```python
from build123d import *

# Parameters (mm, degrees)
ESQUISSE1_W             = 100
ESQUISSE1_H             = 100
BOSS_EXTRU_1_DEPTH      = 5
ESQUISSE2_W             = 20
ESQUISSE2_H             = 5
ENL_V_MAT_EXTRU_1_DEPTH = 142.509716981
ESQUISSE3_W             = 2.886751346
ESQUISSE3_H             = 18
ENL_V_MAT_EXTRU_2_DEPTH = 142.509716981
ENL_V_MAT_EXTRU_5_DEPTH = 18
ENL_V_MAT_EXTRU_6_DEPTH = 18
ENL_V_MAT_EXTRU_7_DEPTH = 18
ENL_V_MAT_EXTRU_8_DEPTH = 18


with BuildPart() as part:
    # Esquisse1 → Boss.-Extru.1 (new body)
    with BuildSketch(Plane.XY):
        with Locations((-50, -50)):
            Rectangle(ESQUISSE1_W, ESQUISSE1_H)
    extrude(amount=BOSS_EXTRU_1_DEPTH)

    # Esquisse2 → Enlèv. mat.-Extru.1 (cut, through all)
    with BuildSketch(Plane.XY.offset(5)):
        with Locations((-70, -2.5)):
            Rectangle(ESQUISSE2_W, ESQUISSE2_H)
        with Locations((-30, -2.5)):
            Rectangle(ESQUISSE2_W, ESQUISSE2_H)
        with Locations((-30, -97.5)):
            Rectangle(ESQUISSE2_W, ESQUISSE2_H)
        with Locations((-70, -97.5)):
            Rectangle(ESQUISSE2_W, ESQUISSE2_H)
    extrude(amount=-ENL_V_MAT_EXTRU_1_DEPTH, mode=Mode.SUBTRACT)

    # Esquisse3 → Enlèv. mat.-Extru.2 (cut, through all)
    with BuildSketch(Plane.XY.offset(5)):
        with Locations((-98.556624327, -32)):
            Rectangle(ESQUISSE3_W, ESQUISSE3_H)
        with Locations((-98.556624327, -68)):
            Rectangle(ESQUISSE3_W, ESQUISSE3_H)
        with Locations((-1.443375673, -68)):
            Rectangle(ESQUISSE3_W, ESQUISSE3_H)
        with Locations((-1.443375673, -32)):
            Rectangle(ESQUISSE3_W, ESQUISSE3_H)
    extrude(amount=-ENL_V_MAT_EXTRU_2_DEPTH, mode=Mode.SUBTRACT)

    # Esquisse5 → Enlèv. mat.-Extru.5 (cut)
    with BuildSketch(Plane.XZ.offset(59)):
        Polygon((-97.113248654, 0), (-97.113248654, 5), (-94.226497308, 0), align=None)
    extrude(amount=ENL_V_MAT_EXTRU_5_DEPTH, mode=Mode.SUBTRACT)

    # Esquisse6 → Enlèv. mat.-Extru.6 (cut)
    with BuildSketch(Plane(origin=(0, -41, 0), x_dir=(1, 0, 0), z_dir=(0, 1, 0))):
        Polygon((-97.113248654, 0), (-97.113248654, -5), (-94.226497308, 0), align=None)
    extrude(amount=ENL_V_MAT_EXTRU_6_DEPTH, mode=Mode.SUBTRACT)

    # Esquisse7 → Enlèv. mat.-Extru.7 (cut)
    with BuildSketch(Plane.XZ.offset(59)):
        Polygon((-2.886751346, 0), (-2.886751346, 5), (-5.773502692, 0), align=None)
    extrude(amount=ENL_V_MAT_EXTRU_7_DEPTH, mode=Mode.SUBTRACT)

    # Esquisse8 → Enlèv. mat.-Extru.8 (cut)
    with BuildSketch(Plane.XZ.offset(23)):
        Polygon((-2.886751346, 0), (-2.886751346, 5), (-5.773502692, 0), align=None)
    extrude(amount=ENL_V_MAT_EXTRU_8_DEPTH, mode=Mode.SUBTRACT)


solid = part.part
```
Verification items for the finished model (mm, model axes). A direction names the side the tool comes from. Coordinates: 2 decimals unless noted, no trailing zeros. Loops run counter-clockwise (first coordinate to the right, second up) from the corner with the lowest first, then second, coordinate; pieces in that order, holes last. Notation, with made-up numbers: (36.5, 77.25) -> (47.5, 77.25) arc R10 ccw to (47.5, 96.25) -> close; hole circle Ø2 at (14, 83). An arc over 180 degrees is marked (long way). Answer in a Markdown table with one row per item.
1) Scan lines: line 1 along Y through (x, z) = (-95, 0.75); line 2 along Y through (x, z) = (-75.5, 4); line 3 along X through (y, z) = (-27.5, 1.75). Record each from-to range of solid material in increasing order. Write a range as from..to.
The answers:
| item | result |
|---|---|
| line 1 | y = -100..-77, -59..-41, -23..0 |
| line 2 | y = -95..-5 |
| line 3 | x = -95.24..-4.76 |
2) Depth check by flat-ended pin: P1, Ø1.5, axis at x = -29, z = 1.5, coming from the +Y side. Enter the tip coordinate at first touch or a pass-through.
The answers:
| item | result |
|---|---|
| P1 | stops at y = -5 |
3) Section check B-B (x = -34). Record the cut outline in (y, z), and give its area (3 significant figures).
The answers:
| item | result |
|---|---|
| outline | (-95, 0) -> (-5, 0) -> (-5, 5) -> (-95, 5) -> close |
| area | 450 mm2 |
4) Draft check along X on faces 1 (the face through (0, -89, 2)), 2 (the face through (-95.69, -32.126, 2.535)), 3 (the face through (-40, -98, 3)). Enter one of: released by +X, released by -X, zero draft, split by the parting line, or undercut.
The answers:
| item | result |
|---|---|
| face 1 | released by +X |
| face 2 | released by -X |
| face 3 | undercut |
5) Access from +Z, -Z, +X, -X, +Y, -Y to the whole of each face (thin tool, end or side, straight path). Record for faces 4 (the face through (-2, -77, 3)), 5 (the face through (-90, -100, 2)), 6 (the face through (-98, -41, 3)), 7 (the face through (-40, -3, 3)), 8 (the face through (-80, -98, 3)).
The answers:
| item | result |
|---|---|
| face 4 | -Z, +X |
| face 5 | +Z, -Z, +X, -X, -Y |
| face 6 | -Z, -X |
| face 7 | +Z, -Z, +Y |
| face 8 | +Z, -Z, -Y |
6) Section check A-A (y = -32.5). Record the cut outline in (x, z), and give its area (3 significant figures).
The answers:
| item | result |
|---|---|
| outline | (-97.11, 5) -> (-94.23, 0) -> (-5.77, 0) -> (-2.89, 5) -> close |
| area | 457 mm2 |
